Verification items for the finished model (mm, model axes). Give positions to 0.01 mm unless a question says otherwise; leave off trailing zeros. Order: outer loops, then holes, each group sorted by start corner. A loop starts at its lowest first (then second) coordinate and runs counter-clockwise, first axis right, second up. Notation, with made-up numbers: M 75.5,-27.75 L 108.5,-27.75 A22 ccw 108.5,-1.75 Z; hole C -22.5,89.5 d7. An arc over 180 degrees is marked long. Answer as a JSON object with one key per item and string values.
```python
from build123d import *

# Parameters (mm, degrees)
SKETCH1_R           = 1.499690954
BOSS_EXTRUDE2_DEPTH = 5
CUT_EXTRUDE3_DEPTH  = 2.5


with BuildPart() as part:
    # Sketch1 → Boss-Extrude2 (new body)
    with BuildSketch(Plane(origin=(0, 0, 0), x_dir=(1, 0, 0), z_dir=(0, 1, 0))):
        Polygon((0, 0), (56.773285815, 82.321285326), (60.754153273, 79.57586019), (3.980867458, -2.745425136), align=None)
        with Locations(Location((3.182714522, 0.391186569, 0), (0, 0, 270))):
            Circle(SKETCH1_R, mode=Mode.SUBTRACT)
    extrude(amount=BOSS_EXTRUDE2_DEPTH)

    # Sketch2 → Cut-Extrude3 (cut)
    with BuildSketch(Plane(origin=(0, 5, 0), x_dir=(1, 0, 0), z_dir=(0, 1, 0))):
        with BuildLine():
            Line((6.700962503, 1.19871368), (3.980867458, -2.745425136))
            Line((3.980867458, -2.745425136), (0, 0))
            Line((0, 0), (2.720095045, 3.944138817))
            ThreePointArc((2.720095045, 3.944138817), (5.279124937, 3.395890894), (6.700962503, 1.19871368))
        make_face()
    extrude(amount=-CUT_EXTRUDE3_DEPTH, mode=Mode.SUBTRACT)


solid = part.part
```
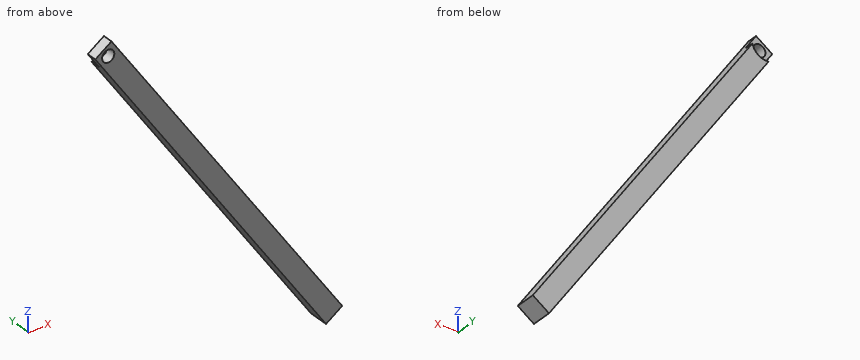
Q1. Section check A-A on y = 1.65. Record the cut outline in (x, z), then the cut area to 3 significant figures.
Resolved:
{"outline": "M 0,0 L 56.77,-82.32 L 60.75,-79.58 L 3.98,2.75 Z; hole C 3.18,-0.39 d3", "area": "477 mm²"}
Q2. Material ranges on L1, parallel to X at y = 2.7, z = -31.5; L2, parallel to Z at x = 20.5, y = 4.3 (3 decimals); L3, parallel to X at y = 0.75, z = -67, recorded low to high.
Resolved:
{"L1": "x = 21.72 to 27.6", "L2": "z = -29.725 to -21.207", "L3": "x = 46.21 to 52.08"}
Q3. Section check B-B on x = 48. Record the cut outline in (y, z), then the cut area to 3 significant figures.
Resolved:
{"outline": "M 0,-69.6 L 5,-69.6 L 5,-61.08 L 0,-61.08 Z", "area": "42.6 mm²"}
Q4. Section check C-C on z = -76. Record the cut outline in (x, y), then the cut area to 3 significant figures.
Resolved:
{"outline": "M 52.41,0 L 58.29,0 L 58.29,5 L 52.41,5 Z", "area": "29.4 mm²"}
Q5. Gauge pin test, flat ends, axial feed: pin 1 Ø5 at (x, z) = (3.18, -0.39) entering from +Y; pin 2 Ø1 at (x, y) = (30, 4) entering from -Z (3 decimals); pin 3 Ø1 at (x, y) = (34.5, 2.5) entering from +Z; pin 4 Ø5 at (x, z) = (34, -55.5) entering from +Y. Record the tip position at first contact, or that the pin passes through.
Resolved:
{"pin 1": "stops at y = 2.5", "pin 2": "stops at z = -44.225", "pin 3": "stops at z = -40.78", "pin 4": "passes through"}
